```python
from build123d import *

# Parameters (mm, degrees)
SKETCH1_W                    = 40
SKETCH1_H                    = 60
SKETCH1_R                    = 3.325
BOSS_EXTRUDE1_DEPTH          = 10
ESQUISSE1_W                  = 10
ESQUISSE1_H                  = 3
BOSS_EXTRU_1_DEPTH           = 10
ESQUISSE2_W                  = 10
ESQUISSE2_H                  = 3
BOSS_EXTRU_2_DEPTH           = 10
ENL_V_MAT_EXTRU_1_DEPTH      = 66.184353951
ENL_V_MAT_EXTRU_1_DEPTH_BACK = 66.184353951
ESQUISSE3_R                  = 1.65


with BuildPart() as part:
    # Sketch1 → Boss-Extrude1 (new body)
    with BuildSketch(Plane.XY):
        Rectangle(SKETCH1_W, SKETCH1_H)
        with Locations((0, 18.11)):
            Circle(SKETCH1_R, mode=Mode.SUBTRACT)
    extrude(amount=BOSS_EXTRUDE1_DEPTH)

    # Esquisse1 → Boss.-Extru.1 (add)
    with BuildSketch(Plane(origin=(20, 0, 0), x_dir=(0, 0, -1), z_dir=(1, 0, 0))):
        with Locations((-5, 28.5)):
            Rectangle(ESQUISSE1_W, ESQUISSE1_H)
        with Locations((-5, -28.5)):
            Rectangle(ESQUISSE1_W, ESQUISSE1_H)
    extrude(amount=BOSS_EXTRU_1_DEPTH)

    # Esquisse2 → Boss.-Extru.2 (add)
    with BuildSketch(Plane.ZY.offset(20)):
        with Locations((5, 28.5)):
            Rectangle(ESQUISSE2_W, ESQUISSE2_H)
        with Locations((5, -28.5)):
            Rectangle(ESQUISSE2_W, ESQUISSE2_H)
    extrude(amount=BOSS_EXTRU_2_DEPTH)

    # Esquisse3 → Enlèv. mat.-Extru.1 (cut, two sides: drawn at the far end of the back side and taken through both)
    with BuildSketch(Plane.XZ.offset(-27).offset(-ENL_V_MAT_EXTRU_1_DEPTH_BACK)):
        with Locations((-25, 5)):
            Circle(ESQUISSE3_R)
        with Locations((25, 5)):
            Circle(ESQUISSE3_R)
    extrude(amount=ENL_V_MAT_EXTRU_1_DEPTH + ENL_V_MAT_EXTRU_1_DEPTH_BACK, mode=Mode.SUBTRACT)


solid = part.part
```
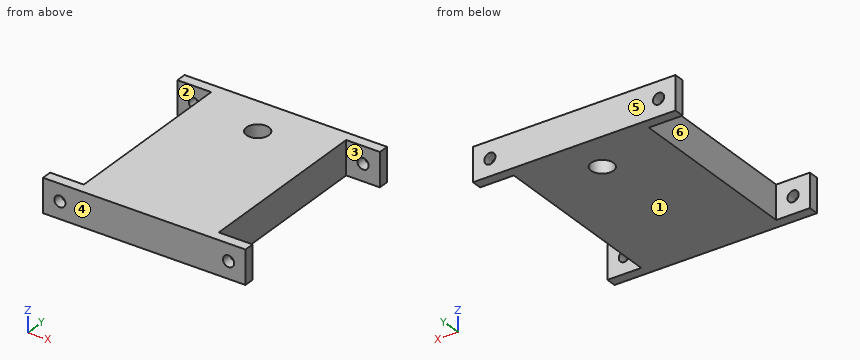
Work out the finished part from the listing and answer in its coordinate system (mm). Face numbers are marked on the shaded views. A direction names the side the tool comes from. Round coordinates to 2 decimals unless told otherwise and drop trailing zeros. Write each loop counter-clockwise with the first axis right and the second up, starting at its lowest first coordinate (ties: lowest second). Pieces come first, ordered by that corner, then holes.
1) A cutting plane is placed at C-C on x = 25. Determine the outline of the cut face in (y, z), and give its area (3 significant figures).
2) A cutting plane is placed at D-D on x = 0. Determine the outline of the cut face in (y, z) (3 decimals).
3) A cutting plane is placed at B-B on y = 18.11. Determine the outline of the cut face in (x, z) (3 decimals).
4) Determine the mould class of the marked faces 4, 5 and 6 for opening direction Y: pulls with the +Y half, pulls with the -Y half, needs draft (parallel to the pull), parting line crosses it, or undercut.
5) A cutting plane is placed at A-A on z = 5. Give the number of separate pieces and of enclosed holes in the cut face, and give its area (3 significant figures).
6) Consider probe 1 along X at (y, z) = (-29.4, 5); probe 2 along Y at (x, z) = (-27, 4.5); probe 3 along Y at (x, z) = (0, 8.25) (3 decimals). Determine where each line is inside the solid, lowest interval first.
7) Which of the six approach directions +Z, -Z, +X, -X, +Y, -Y give full straight-line access (tool end or side, diameter ignored) to the marked faces 1, 2 and 3?
8) Flat-ended cylindrical pins translate along their axes: P1, Ø3, axis at x = 25, z = 5, coming from the +Y side; P2, Ø5, axis at y = 11, z = 4, coming from the -X side. Find the tip coordinate at first contact, or state that the pin passes through.
Entries:
1. outline: (-30, 0) - (-27, 0) - (-27, 3.35) - (-30, 3.35) - close; (-30, 6.65) - (-27, 6.65) - (-27, 10) - (-30, 10) - close; (27, 0) - (30, 0) - (30, 3.35) - (27, 3.35) - close; (27, 6.65) - (30, 6.65) - (30, 10) - (27, 10) - close
1. area: 40.2 mm2
2. outline: (-30, 0) - (14.785, 0) - (14.785, 10) - (-30, 10) - close; (21.435, 0) - (30, 0) - (30, 10) - (21.435, 10) - close
3. outline: (-20, 0) - (-3.325, 0) - (-3.325, 10) - (-20, 10) - close; (3.325, 0) - (20, 0) - (20, 10) - (3.325, 10) - close
4. face 4: pulls with the -Y half
4. face 5: pulls with the +Y half
4. face 6: undercut
5. separate pieces: 5
5. enclosed holes: 1
5. area: 2,450 mm2
6. probe 1: x = -30 to -26.65, -23.35 to 23.35, 26.65 to 30
6. probe 2: y = -30 to -27, 27 to 30
6. probe 3: y = -30 to 14.785, 21.435 to 30
7. face 1: -Z, +X, -X, +Y, -Y
7. face 2: +Z, -Z, -X
7. face 3: +Z, -Z, +X
8. P1: passes through
8. P2: stops at x = -20
